```python
from build123d import *
from OCP.BRepFilletAPI import BRepFilletAPI_MakeChamfer

# Parameters (mm, degrees)
EXTRUDE1_DEPTH      = 4.826
EXTRUDE1_DEPTH_BACK = 4.826
SKETCH10_R          = 1.8
SKETCH10_W          = 1.233836604
SKETCH10_H          = 1.6931216
EXTRUDE5_DEPTH      = 16.428369203
SKETCH6_W           = 0.8
SKETCH6_H           = 0.52
EXTRUDE6_DEPTH      = 13
EXTRUDE7_START      = -0.52
EXTRUDE7_DEPTH      = 0.52
CHAMFER1_SIZE       = 0.254
SKETCH12_W          = 7.379682426
SKETCH12_H          = 2.736118788
EXTRUDE8_DEPTH      = 0.254
SKETCH13_W          = 7.379682426
SKETCH13_H          = 2.736118788
EXTRUDE9_DEPTH      = 0.254
CHAMFER2_SIZE       = 0.508
CHAMFER2_SIZE2      = 0.91645626
CHAMFER3_SIZE       = 0.2032
CHAMFER3_SIZE2      = 0.366582504
CHAMFER3_SIZE2_2    = 0.605677555
CHAMFER3_SIZE2_3    = 0.557834937
EXTRUDE10_DEPTH     = 1.016


with BuildPart() as part:
    # Sketch2 → Extrude1 (new, two sides)
    with BuildSketch(Plane(origin=(0, 0, 0), x_dir=(0, 0, -1), z_dir=(1, 0, 0))) as extrude1_sk:
        Polygon((14.3005, 0), (-1.0795, 0), (-1.0795, 4.5), (7.124012877, 4.5), (7.8005, 1.3), (14.3005, 1.3), align=None)
    extrude(amount=EXTRUDE1_DEPTH)
    extrude(extrude1_sk.sketch, amount=-EXTRUDE1_DEPTH_BACK)

    # Sketch10 → Extrude5 (cut, through all)
    with BuildSketch(Plane(origin=(0, 1.3, 0), x_dir=(1, 0, 0), z_dir=(0, 1, 0))):
        with Locations(Location((0, 11.3505, 0), (0, 0, 270))):
            Circle(SKETCH10_R)
        with Locations((-4.209081698, 11.892729701)):
            Rectangle(SKETCH10_W, SKETCH10_H)
        with Locations((4.209081698, 11.892729701)):
            Rectangle(SKETCH10_W, SKETCH10_H)
    extrude(amount=-EXTRUDE5_DEPTH, mode=Mode.SUBTRACT)

    # Sketch6 → Extrude6 (add)
    with BuildSketch(Plane.XY.offset(1.0795)):
        with Locations((2.54, 2.25)):
            Rectangle(SKETCH6_W, SKETCH6_H)
        with Locations((-2.54, 2.25)):
            Rectangle(SKETCH6_W, SKETCH6_H)
        with Locations((0, 2.25)):
            Rectangle(SKETCH6_W, SKETCH6_H)
    extrude(amount=EXTRUDE6_DEPTH)

    # Sketch11 → Extrude7 (add)
    with BuildSketch(Plane(origin=(0, 2.51, 0), x_dir=(1, 0, 0), z_dir=(0, 1, 0)).offset(EXTRUDE7_START)):
        Polygon((-2.94, -2.0475), (-3.29, -2.0475), (-3.29, -3.5395), (-3.2004, -3.5395), (-3.2004, -3.7747), (-2.94, -4.0795), align=None)
        Polygon((-1.79, -2.0475), (-2.14, -2.0475), (-2.14, -4.0795), (-1.8796, -3.7747), (-1.8796, -3.5395), (-1.79, -3.5395), align=None)
        Polygon((-0.4, -2.0475), (-0.75, -2.0475), (-0.75, -3.5395), (-0.6604, -3.5395), (-0.6604, -3.7747), (-0.4, -4.0795), align=None)
        Polygon((0.75, -2.0475), (0.4, -2.0475), (0.4, -4.0795), (0.6604, -3.7747), (0.6604, -3.5395), (0.75, -3.5395), align=None)
        Polygon((2.14, -2.0475), (1.79, -2.0475), (1.79, -3.5395), (1.8796, -3.5395), (1.8796, -3.7747), (2.14, -4.0795), align=None)
        Polygon((3.29, -2.0475), (2.94, -2.0475), (2.94, -4.0795), (3.2004, -3.7747), (3.2004, -3.5395), (3.29, -3.5395), align=None)
    extrude(amount=EXTRUDE7_DEPTH)

    # Chamfer1
    chamfer1_edges = [part.edges().sort_by_distance(p)[0] for p in [
        (-2.14, 2.25, 14.0795),
        (-2.94, 2.25, 14.0795),
        (2.94, 2.25, 14.0795),
        (2.14, 2.25, 14.0795),
        (0.4, 2.25, 14.0795),
        (-0.4, 2.25, 14.0795),
    ]]
    chamfer(chamfer1_edges, length=CHAMFER1_SIZE)

    # Sketch12 → Extrude8 (cut)
    with BuildSketch(Plane.ZY.offset(4.826)):
        with Locations((-11.490341213, 1.368059394)):
            Rectangle(SKETCH12_W, SKETCH12_H)
    extrude(amount=-EXTRUDE8_DEPTH, mode=Mode.SUBTRACT)

    # Sketch13 → Extrude9 (cut)
    with BuildSketch(Plane(origin=(4.826, 0, 0), x_dir=(0, 0, -1), z_dir=(1, 0, 0))):
        with Locations((11.490341213, 1.368059394)):
            Rectangle(SKETCH13_W, SKETCH13_H)
    extrude(amount=-EXTRUDE9_DEPTH, mode=Mode.SUBTRACT)

    # Chamfer2: one chamfer whose edges measure the first distance from different faces: ONE call of the kernel's chamfer builder (chamfer() names one face for all edges)
    chamfer2_edges_1 = [part.edges().sort_by_distance(p)[0] for p in [
        (-4.826, 4.5, -3.022256439),
    ]]
    chamfer2_side_1 = [part.faces().sort_by_distance(p)[0] for p in [
        (-4.826, 2.217055195, -3.243165334),
    ]]
    chamfer2_edges_2 = [part.edges().sort_by_distance(p)[0] for p in [
        (4.826, 4.5, -3.022256439),
    ]]
    chamfer2_side_2 = [part.faces().sort_by_distance(p)[0] for p in [
        (4.826, 2.217055195, -3.243165334),
    ]]
    chamfer2 = BRepFilletAPI_MakeChamfer(part.part.solid().wrapped)
    for e in chamfer2_edges_1:
        chamfer2.Add(CHAMFER2_SIZE, CHAMFER2_SIZE2, e.wrapped, chamfer2_side_1[0].wrapped)  # the first distance lies on this face
    for e in chamfer2_edges_2:
        chamfer2.Add(CHAMFER2_SIZE, CHAMFER2_SIZE2, e.wrapped, chamfer2_side_2[0].wrapped)  # the first distance lies on this face
    add(Compound.cast(chamfer2.Shape()), mode=Mode.REPLACE)

    # Chamfer3: one chamfer whose edges measure the first distance from different faces: ONE call of the kernel's chamfer builder (chamfer() names one face for all edges)
    chamfer3_edges_1 = [part.edges().sort_by_distance(p)[0] for p in [
        (0, 4.5, 1.0795),
    ]]
    chamfer3_side_1 = [part.faces().sort_by_distance(p)[0] for p in [
        (0, 4.5, -3.022256439),
    ]]
    chamfer3_edges_2 = [part.edges().sort_by_distance(p)[0] for p in [
        (-4.36777187, 4.246, 1.0795),
    ]]
    chamfer3_side_2 = [part.faces().sort_by_distance(p)[0] for p in [
        (-4.368765147, 4.245449417, -3.049162718),
    ]]
    chamfer3_edges_3 = [part.edges().sort_by_distance(p)[0] for p in [
        (4.36777187, 4.246, 1.0795),
    ]]
    chamfer3_side_3 = [part.faces().sort_by_distance(p)[0] for p in [
        (4.368765147, 4.245449417, -3.049162718),
    ]]
    chamfer3_edges_4 = [part.edges().sort_by_distance(p)[0] for p in [
        (0, 4.5, -7.124012877),
    ]]
    chamfer3_side_4 = [part.faces().sort_by_distance(p)[0] for p in [
        (0, 4.5, -3.022256439),
    ]]
    chamfer3_edges_5 = [part.edges().sort_by_distance(p)[0] for p in [
        (-4.36777187, 4.246, -7.177709043),
    ]]
    chamfer3_side_5 = [part.faces().sort_by_distance(p)[0] for p in [
        (-4.368765147, 4.245449417, -3.049162718),
    ]]
    chamfer3_edges_6 = [part.edges().sort_by_distance(p)[0] for p in [
        (4.36777187, 4.246, -7.177709043),
    ]]
    chamfer3_side_6 = [part.faces().sort_by_distance(p)[0] for p in [
        (4.368765147, 4.245449417, -3.049162718),
    ]]
    chamfer3 = BRepFilletAPI_MakeChamfer(part.part.solid().wrapped)
    for e in chamfer3_edges_1:
        chamfer3.Add(CHAMFER3_SIZE, CHAMFER3_SIZE2, e.wrapped, chamfer3_side_1[0].wrapped)  # the first distance lies on this face
    for e in chamfer3_edges_2:
        chamfer3.Add(CHAMFER3_SIZE, CHAMFER3_SIZE2, e.wrapped, chamfer3_side_2[0].wrapped)  # the first distance lies on this face
    for e in chamfer3_edges_3:
        chamfer3.Add(CHAMFER3_SIZE, CHAMFER3_SIZE2, e.wrapped, chamfer3_side_3[0].wrapped)  # the first distance lies on this face
    for e in chamfer3_edges_4:
        chamfer3.Add(CHAMFER3_SIZE, CHAMFER3_SIZE2_2, e.wrapped, chamfer3_side_4[0].wrapped)  # the first distance lies on this face
    for e in chamfer3_edges_5:
        chamfer3.Add(CHAMFER3_SIZE, CHAMFER3_SIZE2_3, e.wrapped, chamfer3_side_5[0].wrapped)  # the first distance lies on this face
    for e in chamfer3_edges_6:
        chamfer3.Add(CHAMFER3_SIZE, CHAMFER3_SIZE2_3, e.wrapped, chamfer3_side_6[0].wrapped)  # the first distance lies on this face
    add(Compound.cast(chamfer3.Shape()), mode=Mode.REPLACE)

    # Sketch15 → Extrude10 (add)
    with BuildSketch(Plane.XY.offset(4.0795)):
        with BuildLine():
            Line((-2.14, 2.51), (-2.94, 2.51))
            ThreePointArc((-2.94, 2.51), (-3.017074418, 2.25), (-2.94, 1.99))
            Line((-2.94, 1.99), (-2.14, 1.99))
            ThreePointArc((-2.14, 1.99), (-2.062925582, 2.25), (-2.14, 2.51))
        make_face()
    extrude(amount=-EXTRUDE10_DEPTH)


solid = part.part
```
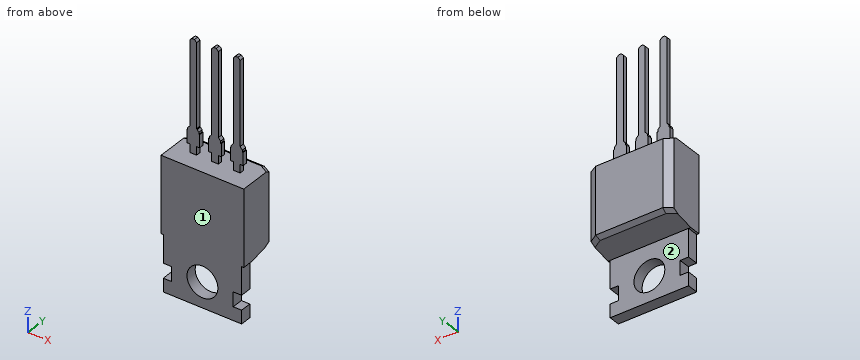
Read the model definition and answer for the solid it produces. Units are mm, in the model's axes. Face numbers are marked on the shaded views. A direction names the side the tool comes from. Coordinates: 2 decimals unless noted, no trailing zeros. Loops run counter-clockwise (first coordinate to the right, second up) from the corner with the lowest first, then second, coordinate; pieces in that order, holes last.
(1) The part is cut by section D-D (y = 1.7). Determine the outline of the cut face in (x, z).
Solution:
outline: (-4.83, -7.72) - (4.83, -7.72) - (4.83, 1.08) - (-4.83, 1.08) - close
(2) The part is cut by section A-A (z = 7.25). Determine the outline of the cut face in (x, y).
Solution:
outline: (-2.94, 1.99) - (-2.14, 1.99) - (-2.14, 2.51) - (-2.94, 2.51) - close; (-0.4, 1.99) - (0.4, 1.99) - (0.4, 2.51) - (-0.4, 2.51) - close; (2.14, 1.99) - (2.94, 1.99) - (2.94, 2.51) - (2.14, 2.51) - close
(3) The part is cut by section B-B (x = 1.5). Determine the outline of the cut face in (y, z), and give its area (3 significant figures).
Solution:
outline: (0, -14.3) - (1.3, -14.3) - (1.3, -12.35) - (0, -12.35) - close; (0, -10.36) - (1.3, -10.36) - (1.3, -7.8) - (3.91, -7.25) - (4.5, -6.92) - (4.5, 0.88) - (4.13, 1.08) - (0, 1.08) - close
area: 44.6 mm2
(4) Consider line 1 along Z through (x, y) = (4, 0.3); line 2 along Y through (x, z) = (-2.75, 6); line 3 along Z through (x, y) = (4, 3.65). Determine where each line is inside the solid, lowest interval first.
Solution:
line 1: z = -14.3 to -12.74, -11.05 to 1.08
line 2: y = 1.99 to 2.51
line 3: z = -7.3 to 1.08
(5) The part is cut by section C-C (z = -8.75). Determine the outline of the cut face in (x, y).
Solution:
outline: (-4.57, 0) - (4.57, 0) - (4.57, 1.3) - (-4.57, 1.3) - close
(6) Flat-ended cylindrical pins translate along their axes: pin 1 Ø2 at (x, z) = (0, -11.35) entering from -Y; pin 2 Ø0.6 at (y, z) = (2.5, 2.5) entering from +X; pin 3 Ø0.6 at (y, z) = (0.5, -9.5) entering from +X; pin 4 Ø1.6 at (x, z) = (2.5, 8.5) entering from +Y. Find the tip coordinate at first contact, or state that the pin passes through.
Solution:
pin 1: passes through
pin 2: stops at x = 3.29
pin 3: stops at x = 4.57
pin 4: stops at y = 2.51
(7) A tool of negligible diameter and unlimited length cuts with its end or side. For the marked faces 1 and 2, from which of +Z, -Z, +X, -X, +Y, -Y can it reach the whole face along a straight path? Write none if from no direction.
Solution:
face 1: +Z, -Z, +X, -X, -Y
face 2: -Z, +X, -X, +Y
